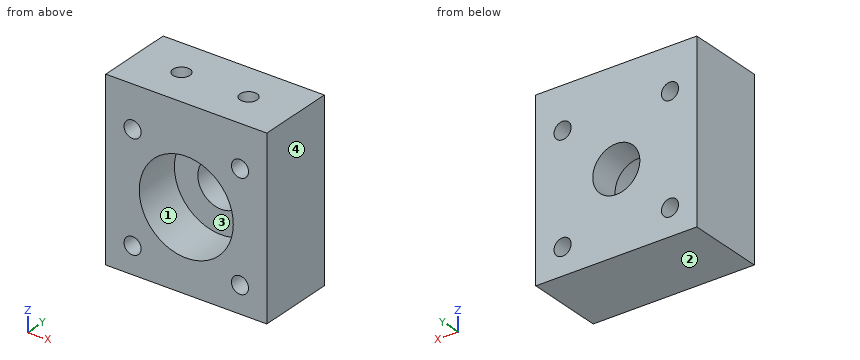
from build123d import *

# Parameters (mm, degrees)
F0_W     = 38.1
F0_H     = 38.1
F0_R     = 5.5626
F1_DEPTH = 18.288
F3_D     = 4.0386
F4_R     = 11.1125
F4_R_2   = 5.5626
F5_DEPTH = 11.176
F6_DEPTH = 3.556
F8_D     = 4.0386
F8_DEPTH = 11.811
F8_TIP   = 1.213317848


with BuildPart() as f1:
    # F0 (on Front) → F1 (new body)
    with BuildSketch(Plane.XZ):
        Rectangle(F0_W, F0_H)
        Circle(F0_R, mode=Mode.SUBTRACT)
    extrude(amount=F1_DEPTH)

    # F3 (through all)
    with Locations(Plane.XZ.offset(18.288)):
        with Locations((-12.7, -12.7), (-12.7, 12.7), (12.7, 12.7), (12.7, -12.7)):
            Hole(F3_D / 2)

    # F4 (on face) → F5 (cut)
    with BuildSketch(Plane.XZ.offset(18.288)):
        Circle(F4_R)
        Circle(F4_R_2, mode=Mode.SUBTRACT)
    extrude(amount=-F5_DEPTH, mode=Mode.SUBTRACT)

    # F6 (add): a face of the model
    f6_faces = [f1.faces().sort_by_distance(p)[0] for p in [
        (0, -9.144, 19.05),
    ]]
    extrude(f6_faces, amount=F6_DEPTH)

    # F8
    with Locations(Plane.XY.offset(22.606)):
        with Locations((-7.9248, -9.144), (7.9502, -9.144)):
            Hole(F8_D / 2, depth=F8_DEPTH)
            with Locations((0, 0, -(F8_DEPTH + F8_TIP / 2))):  # 118° drill point
                Cone(0, F8_D / 2, F8_TIP, mode=Mode.SUBTRACT)


solid = f1.part
The listing builds one solid part. Answer for the finished solid, in the listing's coordinates (mm). Face numbers are marked on the shaded views. Round coordinates to 2 decimals unless told otherwise and drop trailing zeros. Loops run counter-clockwise (first coordinate to the right, second up) from the corner with the lowest first, then second, coordinate; pieces in that order, holes last. Notation, with made-up numbers: M 53,-0.5 L 95,-0.5 A26 ccw 95,20.5 Z; hole C -36.5,48.25 d6. An arc over 180 degrees is marked long. Write each question's results on one line, items separated by ' | '. Start each with the question number.
1) Each of these flat-tipped pins is pushed along its axis until it touches: pin 1 (3.5 mm diameter, centred on x = -12.7, z = -12.7, fed in from -Y); pin 2 (4.5 mm diameter, centred on x = 12.7, z = 12.7, fed in from +Y); pin 3 (11 mm diameter, centred on x = 4.5, z = 1.5, fed in from -Y). Where does it stop, or does it pass through?
2) Determine the mould class of the marked faces 1, 2, 3 and 4 for opening direction Z: pulls with the +Z half, pulls with the -Z half, needs draft (parallel to the pull), parting line crosses it, or undercut.
3) Find section C-C on y = -14. Count the separate pieces of the cut face and the enclosed holes in it, plus the area to 3 significant figures.
4) Find section D-D on x = 0. Write down the section's boundary in (y, z), plus the area to 3 significant figures.
5) Find section A-A on x = -12.7. Write down the section's boundary in (y, z), plus the area to 3 significant figures.
6) Straight lines are drawn through the part: probe 1 along Z at (x, y) = (12.7, -6.5); probe 2 along Z at (x, y) = (0, -14.5); probe 3 along X at (y, z) = (-4.5, 11). For each, find the intervals that lie inside material, in ascending order.
7) Find section B-B on z = -12.7. Write down the section's boundary in (x, y), plus the area to 3 significant figures.
Final values:
1) pin 1: through | pin 2: y = 0 | pin 3: y = -7.11
2) face 1: undercut | face 2: pulls with the -Z half | face 3: undercut | face 4: needs draft
3) separate pieces: 1 | enclosed holes: 5 | area: 1,150 mm²
4) outline: M -18.29,-19.05 L 0,-19.05 L 0,-5.56 L -7.11,-5.56 L -7.11,-11.11 L -18.29,-11.11 Z; M -18.29,11.11 L -7.11,11.11 L -7.11,5.56 L 0,5.56 L 0,22.61 L -18.29,22.61 Z | area: 434 mm²
5) outline: M -18.29,-19.05 L 0,-19.05 L 0,-14.72 L -18.29,-14.72 Z; M -18.29,-10.68 L 0,-10.68 L 0,10.68 L -18.29,10.68 Z; M -18.29,14.72 L 0,14.72 L 0,22.61 L -18.29,22.61 Z | area: 614 mm²
6) probe 1: -19.05 to -14.72, -10.68 to 10.68, 14.72 to 22.61 | probe 2: -19.05 to -11.11, 11.11 to 22.61 | probe 3: -19.05 to -13.79, -11.61 to 11.61, 13.79 to 19.05
7) outline: M -19.05,-18.29 L -14.72,-18.29 L -14.72,0 L -19.05,0 Z; M -10.68,-18.29 L 10.68,-18.29 L 10.68,0 L -10.68,0 Z; M 14.72,-18.29 L 19.05,-18.29 L 19.05,0 L 14.72,0 Z | area: 549 mm²
